```python
from build123d import *

# Parameters (mm, degrees)
SKETCH_1_W               = 100
SKETCH_1_H               = 42
EXTRUDE_1_DEPTH          = 6
SKETCH_2_W               = 200
SKETCH_2_H               = 6
EXTRUDE_2_DEPTH          = 79
SKETCH_3_R               = 7
CUT_EXTRUDE_1_DEPTH      = 133.70267518
SKETCH_4_W               = 148
SKETCH_4_H               = 280
EXTRUDE_3_DEPTH          = 10
SKETCH_6_W               = 148
SKETCH_6_H               = 10
EXTRUDE_4_DEPTH          = 325
SKETCH_7_W               = 148
SKETCH_7_H               = 380
EXTRUDE_5_DEPTH          = 10
SKETCH_8_W               = 10
SKETCH_8_H               = 50
EXTRUDE_6_DEPTH          = 50
CUT_EXTRUDE_2_DEPTH      = 517.861683625
SKETCH_10_W              = 260
SKETCH_10_H              = 325
SKETCH_10_R              = 120
EXTRUDE_7_DEPTH          = 10
PATTERN_LINEAR_1_COUNT   = 2
PATTERN_LINEAR_1_PITCH   = 66
SKETCH_12_R              = 120
SKETCH_12_R_2            = 80
EXTRUDE_9_DEPTH          = 148
SKETCH_13_W              = 36
SKETCH_13_H              = 10
EXTRUDE_10_DEPTH         = 50
EXTRUDE_START            = -14
SKETCH_14_R              = 80
SKETCH_14_R_2            = 65
EXTRUDE_11_DEPTH         = 14
SKETCH_15_R              = 65
SKETCH_15_R_2            = 45
EXTRUDE_12_DEPTH         = 5
SKETCH_17_R              = 120
SKETCH_17_R_2            = 45
EXTRUDE_13_DEPTH         = 14
SKETCH_18_R              = 80
SKETCH_18_R_2            = 65
EXTRUDE_14_DEPTH         = 14
SKETCH_19_R              = 65
SKETCH_19_R_2            = 25
EXTRUDE_15_DEPTH         = 5
EXTRUDE_START_2          = 14
SKETCH_20_R              = 120
SKETCH_20_R_2            = 25
EXTRUDE_16_DEPTH         = 14
SKETCH_27_R              = 8.5
CUT_EXTRUDE_4_DEPTH      = 10
SKETCH_28_R              = 5
CUT_EXTRUDE_5_DEPTH      = 25
CUT_EXTRUDE_START        = -25
SKETCH_29_R              = 5
CUT_EXTRUDE_6_DEPTH      = 25
PATTERN_CIRCULAR_2_COUNT = 8


with BuildPart() as part:
    # Sketch 1 → Extrude 1 (new body)
    with BuildSketch(Plane(origin=(0, 0, 0), x_dir=(1, 0, 0), z_dir=(0, 1, 0))):
        with Locations((50, 21)):
            Rectangle(SKETCH_1_W, SKETCH_1_H)
    extrude(amount=EXTRUDE_1_DEPTH)

    # Sketch 2 → Extrude 2 (add)
    with BuildSketch(Plane(origin=(0, 0, 0), x_dir=(1, 0, 0), z_dir=(0, 1, 0))):
        with Locations((0, 34)):
            Rectangle(SKETCH_2_W, SKETCH_2_H)
        with Locations((0, 8)):
            Rectangle(SKETCH_2_W, SKETCH_2_H)
    extrude(amount=-EXTRUDE_2_DEPTH)

    # Sketch 3 → Cut-Extrude 1 (cut, through all)
    with BuildSketch(Plane.XY.offset(-5)):
        with Locations((-35, -25)):
            Circle(SKETCH_3_R)
        with BuildLine():
            Line((-44.049345139, -48.304706661), (35, -79))
            Line((35, -79), (-100, -79))
            Line((-100, -79), (-100, 0))
            Line((-100, 0), (-35, 0))
            ThreePointArc((-35, 0), (-59.572521915, -20.396613558), (-44.049345139, -48.304706661))
        make_face()
    extrude(amount=-CUT_EXTRUDE_1_DEPTH, mode=Mode.SUBTRACT)

    # Sketch 4 → Extrude 3 (add)
    with BuildSketch(Plane(origin=(0, -79, 0), x_dir=(-1, 0, 0), z_dir=(0, -1, 0))):
        with Locations((-109, 21)):
            Rectangle(SKETCH_4_W, SKETCH_4_H)
    extrude(amount=EXTRUDE_3_DEPTH)

    # Sketch 6 → Extrude 4 (add)
    with BuildSketch(Plane(origin=(0, -89, 0), x_dir=(-1, 0, 0), z_dir=(0, -1, 0))):
        with Locations((-109, -114)):
            Rectangle(SKETCH_6_W, SKETCH_6_H)
        with Locations((-109, 156)):
            Rectangle(SKETCH_6_W, SKETCH_6_H)
    extrude(amount=EXTRUDE_4_DEPTH)

    # Sketch 7 → Extrude 5 (add)
    with BuildSketch(Plane(origin=(0, -414, 0), x_dir=(-1, 0, 0), z_dir=(0, -1, 0))):
        with Locations((-109, 21)):
            Rectangle(SKETCH_7_W, SKETCH_7_H)
    extrude(amount=EXTRUDE_5_DEPTH)

    # Sketch 8 → Extrude 6 (add)
    with BuildSketch(Plane(origin=(0, -414, 0), x_dir=(1, 0, 0), z_dir=(0, 1, 0))):
        with Locations((76, 186)):
            Rectangle(SKETCH_8_W, SKETCH_8_H)
        with Locations((142, 186)):
            Rectangle(SKETCH_8_W, SKETCH_8_H)
        with Locations((76, -144)):
            Rectangle(SKETCH_8_W, SKETCH_8_H)
        with Locations((142, -144)):
            Rectangle(SKETCH_8_W, SKETCH_8_H)
    extrude(amount=EXTRUDE_6_DEPTH)

    # Sketch 9 → Cut-Extrude 2 (cut, through all)
    with BuildSketch(Plane(origin=(147, 0, 0), x_dir=(0, 0, -1), z_dir=(1, 0, 0))):
        Polygon((211, -364), (181, -364), (211, -394), align=None)
        Polygon((-169, -364), (-139, -364), (-169, -394), align=None)
    extrude(amount=-CUT_EXTRUDE_2_DEPTH, mode=Mode.SUBTRACT)

    # Sketch 10 → Extrude 7 (add)
    with BuildSketch(Plane(origin=(147, 0, 0), x_dir=(0, 0, -1), z_dir=(1, 0, 0))):
        with Locations((21, -251.5)):
            Rectangle(SKETCH_10_W, SKETCH_10_H)
        with Locations((21, -249)):
            Circle(SKETCH_10_R, mode=Mode.SUBTRACT)
    extrude_7 = extrude(amount=-EXTRUDE_7_DEPTH)

    # Pattern Linear 1: Extrude 7 ×2
    with Locations(*[(-i * PATTERN_LINEAR_1_PITCH, 0, 0) for i in range(1, PATTERN_LINEAR_1_COUNT)]):
        add(extrude_7)



with BuildPart() as body_2:
    # Sketch 12 → Extrude 9 (new body)
    with BuildSketch(Plane.ZY.offset(-35)):
        with Locations(Location((-21, -249, 0), (0, 0, 180))):
            Circle(SKETCH_12_R)
        with Locations((-21, -249)):
            Circle(SKETCH_12_R_2, mode=Mode.SUBTRACT)
    extrude(amount=-EXTRUDE_9_DEPTH)


with BuildPart() as part_1:
    add(part.part)

    add(body_2.part)  # Extrude 10 merges body 2
    # Sketch 13 → Extrude 10 (add)
    with BuildSketch(Plane(origin=(0, -414, 0), x_dir=(1, 0, 0), z_dir=(0, 1, 0))):
        with Locations((165, -24)):
            Rectangle(SKETCH_13_W, SKETCH_13_H)
        with Locations((165, 66)):
            Rectangle(SKETCH_13_W, SKETCH_13_H)
        with Locations((53, 66)):
            Rectangle(SKETCH_13_W, SKETCH_13_H)
        with Locations((53, -24)):
            Rectangle(SKETCH_13_W, SKETCH_13_H)
    extrude(amount=EXTRUDE_10_DEPTH)

    # Sketch 14 → Extrude 11 (add)
    with BuildSketch(Plane(origin=(183, 0, 0), x_dir=(0, 0, -1), z_dir=(1, 0, 0)).offset(EXTRUDE_START)):
        with Locations(Location((21, -249, 0), (0, 0, 180))):
            Circle(SKETCH_14_R)
        with Locations((21, -249)):
            Circle(SKETCH_14_R_2, mode=Mode.SUBTRACT)
    extrude(amount=EXTRUDE_11_DEPTH)



with BuildPart() as body_2_2:
    # Sketch 15 → Extrude 12 (new body)
    with BuildSketch(Plane(origin=(183, 0, 0), x_dir=(0, 0, -1), z_dir=(1, 0, 0))):
        with Locations((21, -249)):
            Circle(SKETCH_15_R)
        with Locations((21, -249)):
            Circle(SKETCH_15_R_2, mode=Mode.SUBTRACT)
    extrude(amount=-EXTRUDE_12_DEPTH)


with BuildPart() as part_2:
    add(part_1.part)

    add(body_2_2.part)  # Extrude 13 merges body 2 2
    # Sketch 17 → Extrude 13 (add)
    with BuildSketch(Plane(origin=(183, 0, 0), x_dir=(0, 0, -1), z_dir=(1, 0, 0))):
        with Locations(Location((21, -249, 0), (0, 0, 180))):
            Circle(SKETCH_17_R)
        with Locations((21, -249)):
            Circle(SKETCH_17_R_2, mode=Mode.SUBTRACT)
    extrude(amount=EXTRUDE_13_DEPTH)

    # Sketch 18 → Extrude 14 (add)
    with BuildSketch(Plane.ZY.offset(-35)):
        with Locations((-21, -249)):
            Circle(SKETCH_18_R)
        with Locations(Location((-21, -249, 0), (0, 0, 180))):
            Circle(SKETCH_18_R_2, mode=Mode.SUBTRACT)
    extrude(amount=-EXTRUDE_14_DEPTH)



with BuildPart() as body_2_3:
    # Sketch 19 → Extrude 15 (new body)
    with BuildSketch(Plane.ZY.offset(-35)):
        with Locations(Location((-21, -249, 0), (0, 0, 180))):
            Circle(SKETCH_19_R)
        with Locations((-21, -249)):
            Circle(SKETCH_19_R_2, mode=Mode.SUBTRACT)
    extrude(amount=-EXTRUDE_15_DEPTH)


with BuildPart() as part_3:
    add(part_2.part)

    add(body_2_3.part)  # Extrude 16 merges body 2 3
    # Sketch 20 → Extrude 16 (add)
    with BuildSketch(Plane.ZY.offset(-35).offset(EXTRUDE_START_2)):
        with Locations((-21, -249)):
            Circle(SKETCH_20_R)
        with Locations((-21, -249)):
            Circle(SKETCH_20_R_2, mode=Mode.SUBTRACT)
    extrude(amount=-EXTRUDE_16_DEPTH)

    # Sketch 27 → Cut-Extrude 4 (cut)
    with BuildSketch(Plane(origin=(0, -424, 0), x_dir=(-1, 0, 0), z_dir=(0, -1, 0))):
        with Locations(Location((-109, -144, 0), (0, 0, 90))):
            Circle(SKETCH_27_R)
        with Locations(Location((-164, -144, 0), (0, 0, 90))):
            Circle(SKETCH_27_R)
        with Locations(Location((-54, -144, 0), (0, 0, 90))):
            Circle(SKETCH_27_R)
        with Locations(Location((-54, 186, 0), (0, 0, 90))):
            Circle(SKETCH_27_R)
        with Locations(Location((-109, 186, 0), (0, 0, 90))):
            Circle(SKETCH_27_R)
        with Locations(Location((-164, 186, 0), (0, 0, 90))):
            Circle(SKETCH_27_R)
        with Locations(Location((-54, 111, 0), (0, 0, 90))):
            Circle(SKETCH_27_R)
        with Locations(Location((-54, -69, 0), (0, 0, 90))):
            Circle(SKETCH_27_R)
        with Locations(Location((-54, 21, 0), (0, 0, 90))):
            Circle(SKETCH_27_R)
    extrude(amount=-CUT_EXTRUDE_4_DEPTH, mode=Mode.SUBTRACT)

    # Sketch 28 → Cut-Extrude 5 (cut)
    with BuildSketch(Plane(origin=(197, 0, 0), x_dir=(0, 0, -1), z_dir=(1, 0, 0))):
        with Locations((21, -149)):
            Circle(SKETCH_28_R)
    cut_extrude_5 = extrude(amount=-CUT_EXTRUDE_5_DEPTH, mode=Mode.SUBTRACT)

    # Sketch 29 → Cut-Extrude 6 (cut)
    with BuildSketch(Plane.ZY.offset(-21).offset(CUT_EXTRUDE_START)):
        with Locations(Location((-21, -149, 0), (0, 0, 180))):
            Circle(SKETCH_29_R)
    cut_extrude_6 = extrude(amount=CUT_EXTRUDE_6_DEPTH, mode=Mode.SUBTRACT)

    # Pattern Circular 2: Cut-Extrude 5, Cut-Extrude 6 ×8 about axis
    pattern_circular_2_axis = Axis((0, -249, -21), (1, 0, 0))
    add([cut_extrude_5.rotate(pattern_circular_2_axis, i * 360 / PATTERN_CIRCULAR_2_COUNT) for i in range(1, PATTERN_CIRCULAR_2_COUNT)], mode=Mode.SUBTRACT)
    add([cut_extrude_6.rotate(pattern_circular_2_axis, i * 360 / PATTERN_CIRCULAR_2_COUNT) for i in range(1, PATTERN_CIRCULAR_2_COUNT)], mode=Mode.SUBTRACT)


solid = part_3.part
```
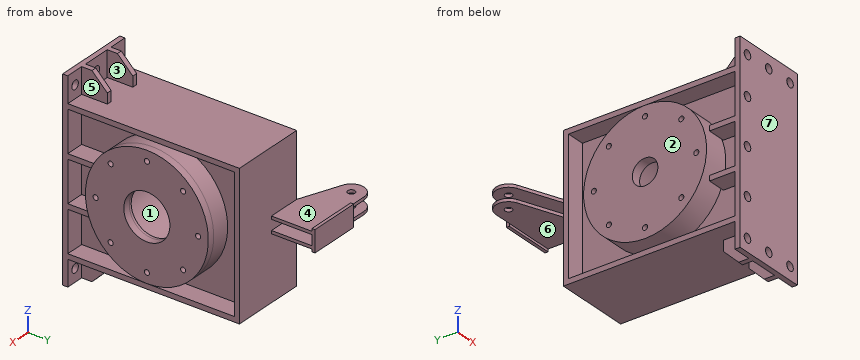
For this review, take the finished solid that the model builds, in its own axes (mm). Face numbers are marked on the shaded views. A direction names the side the tool comes from. Give positions to 0.01 mm unless a question says otherwise; leave off trailing zeros. Order: outer loops, then holes, each group sorted by start corner. A loop starts at its lowest first (then second) coordinate and runs counter-clockwise, first axis right, second up.
1) The part is to be moulded in two halves that separate along Y. For the marked faces 5, 6 and 7, say which applies: released by +Y, released by -Y, zero draft, split by the parting line, or undercut.
2) Insertion check: pin 1 (3 mm diameter, centred on y = -306, z = 69.5, fed in from -X); pin 2 (9 mm diameter, centred on y = -249, z = 79, fed in from -X); pin 3 (6.5 mm diameter, centred on x = -9, z = -35, fed in from +Y). Each pin has a flat end and moves straight along its axis. Give the tip position at first contact, or say it passes through.
3) For the marked faces 1, 2, 3 and 4, list the 3-axis set-ups (+Z, -Z, +X, -X, +Y, -Y) from which the entire face can be reached by the end or side of a thin tool; tool diameter is ignored.
4) Wall thickness on line 1 (Y direction, x = 189.75, z = -21); line 2 (X direction, y = -109.5, z = -86.5); line 3 (Y direction, x = 40.5, z = 26.5): over which ranges is each line inside the solid? List them lowest first.
5) Take a section at A-A (x = 109). Give the boundary of the cut face in (y, z), then the cut area to 3 significant figures.
6) Take a section at B-B (x = -9.5). Give the boundary of the cut face in (y, z).
Derived:
1. face 5: zero draft
1. face 6: undercut
1. face 7: released by -Y
2. pin 1: stops at x = 21
2. pin 2: stops at x = 46
2. pin 3: stops at y = 0
3. face 1: none
3. face 2: +Z, -Z, -X, -Y
3. face 3: +Z, +Y
3. face 4: +Z, +X, -X
4. line 1: y = -369 to -354, -344 to -294, -204 to -154, -144 to -129
4. line 2: x = 71 to 81, 137 to 147
4. line 3: y = -424 to -364, -359.2 to -293.37, -204.63 to -138.8, -89 to -79
5. outline: (-424, -211) - (-414, -211) - (-414, -194.5) - (-424, -194.5) - close; (-424, -177.5) - (-414, -177.5) - (-414, -161) - (-79, -161) - (-79, 119) - (-414, 119) - (-414, 135.5) - (-424, 135.5) - close; (-424, 152.5) - (-414, 152.5) - (-414, 169) - (-424, 169) - close; circle Ø240 at (-249, -21); hole (-414, -151) - (-89, -151) - (-89, 109) - (-414, 109) - close; hole circle Ø160 at (-249, -21)
5. area: 37,900 mm2
6. outline: (-61.72, -37) - (0, -37) - (0, -31) - (-61.72, -31) - close; (-61.72, -11) - (0, -11) - (0, -5) - (-61.72, -5) - close
